Here's how the part is built. I have some questions about the finished solid (model axes, mm). Face numbers are marked on the shaded views. A direction names the side the tool comes from. Round coordinates to 2 decimals unless told otherwise and drop trailing zeros. Loops run counter-clockwise (first coordinate to the right, second up) from the corner with the lowest first, then second, coordinate; pieces in that order, holes last. Notation, with made-up numbers: (-7.75, 85.5) -> (51.25, 85.5) arc R29 ccw to (51.25, 124.5) -> close; hole circle Ø1 at (-10, 18). An arc over 180 degrees is marked (long way). Use CSV: the item, a comma, the result in double quotes. Start each with the question number.
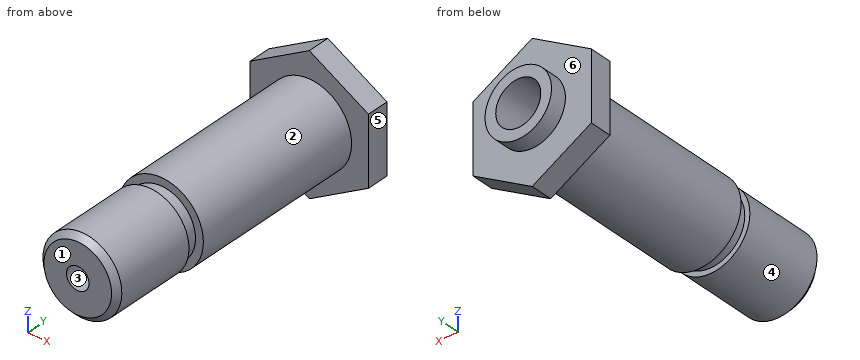
from build123d import *

# Parameters (mm, degrees)
EXTRUDE_1_DEPTH     = 4
SKETCH_2_R          = 5.9
EXTRUDE_2_DEPTH     = 3
SKETCH_3_R          = 7.5
EXTRUDE_3_DEPTH     = 50
SKETCH_4_R          = 4
CUT_EXTRUDE_1_DEPTH = 35
SKETCH_7_R          = 2
CUT_EXTRUDE_2_DEPTH = 58
CHAMFER_1_SIZE      = 1


with BuildPart() as part:
    # Эскиз1 → Бобышка-Вытянуть1 (new body)
    with BuildSketch(Plane(origin=(0, 0, 0), x_dir=(1, 0, 0), z_dir=(0, 1, 0))):
        Polygon((10.5, -6.062177826), (10.5, 6.062177826), (0, 12.124355653), (-10.5, 6.062177826), (-10.5, -6.062177826), (0, -12.124355653), align=None)
    extrude(amount=EXTRUDE_1_DEPTH)

    # Эскиз2 → Бобышка-Вытянуть2 (add)
    with BuildSketch(Plane(origin=(0, 4, 0), x_dir=(1, 0, 0), z_dir=(0, 1, 0))):
        Circle(SKETCH_2_R)
    extrude(amount=EXTRUDE_2_DEPTH)

    # Эскиз3 → Бобышка-Вытянуть3 (add)
    with BuildSketch(Plane.XZ):
        Circle(SKETCH_3_R)
    extrude(amount=EXTRUDE_3_DEPTH)

    # Эскиз4 → Вырез-Вытянуть1 (cut)
    with BuildSketch(Plane(origin=(0, 7, 0), x_dir=(1, 0, 0), z_dir=(0, 1, 0))):
        Circle(SKETCH_4_R)
    extrude(amount=-CUT_EXTRUDE_1_DEPTH, mode=Mode.SUBTRACT)

    # Эскиз6 → Вырез-Повернуть1 (revolve, cut)
    with BuildSketch(Plane(origin=(0, 0, 0), x_dir=(0, 0, -1), z_dir=(1, 0, 0))):
        Polygon((7.5, -50), (7.5, -32), (6.1, -32), (6.1, -34.5), (7, -34.5), (7, -50), align=None)
    revolve(axis=Axis((0, -50.526489701, 0), (0, 1, 0)), mode=Mode.SUBTRACT)

    # Эскиз7 → Вырез-Вытянуть2 (cut, through all)
    with BuildSketch(Plane.XZ.offset(50)):
        Circle(SKETCH_7_R)
    extrude(amount=-CUT_EXTRUDE_2_DEPTH, mode=Mode.SUBTRACT)

    # Фаска1
    chamfer_1_edges = [part.edges().sort_by_distance(p)[0] for p in [
        (0, -50, 7),
    ]]
    chamfer(chamfer_1_edges, length=CHAMFER_1_SIZE)


solid = part.part
Q1. I need wall thicknesses on line 1 along Z through (x, y) = (0, -38.75); line 2 along X through (y, z) = (-23.5, 0); line 3 along Y through (x, z) = (0.5, -3.75). Which ranges of each line are inside material? Lowest first, please.
Q2. I want a section at D-D, the plane z = 8.75. List the corners of the cut face in (x, y) for me.
Q3. If we mould it in two halves opening along X, with no side actions, what happens to the marked faces 1, 2 and 3? For each: pulls with the +X half, pulls with the -X half, needs draft (parallel to the pull), parting line crosses it, or undercut.
Q4. Will these pins go through, and if not, where does the flat tip stop? pin 1 Ø10 at (x, y) = (-5.5, -0.5) entering from +Z; pin 2 Ø5 at (x, y) = (-1.5, -7.5) entering from -Z; pin 3 Ø1 at (y, z) = (-26.5, 4) entering from +X; pin 4 Ø1.5 at (x, y) = (-8.5, -19) entering from +Z (3 decimals).
Q5. For the marked faces 4, 5 and 6, which set-ups out of +Z, -Z, +X, -X, +Y, -Y let a thin tool reach every point of the face, with its end or its side?
Q6. I want a section at B-B, the plane y = 1. List the corners of the cut face in (x, z) for me, then the cut area to 3 significant figures.
Q7. I want a section at C-C, the plane y = -36.5. List the corners of the cut face in (x, z) for me.
Values found:
1,line 1,"-7 to -2, 2 to 7"
1,line 2,"-7.5 to -4, 4 to 7.5"
1,line 3,"-50 to -28"
2,outline,"(-5.84, 0) -> (5.84, 0) -> (5.84, 4) -> (-5.84, 4) -> close"
3,face 1,"needs draft"
3,face 2,"parting line crosses it"
3,face 3,"undercut"
4,pin 1,"z = 11.82"
4,pin 2,"z = -7.5"
4,pin 3,"x = 6.63"
4,pin 4,"through"
5,face 4,"-Y"
5,face 5,"+Z, -Z, +X, +Y, -Y"
5,face 6,"+Y"
6,outline,"(-10.5, -6.06) -> (0, -12.12) -> (10.5, -6.06) -> (10.5, 6.06) -> (0, 12.12) -> (-10.5, 6.06) -> close; hole circle Ø8 at (0, 0)"
6,area,"332 mm2"
7,outline,"circle Ø14 at (0, 0); hole circle Ø4 at (0, 0)"
